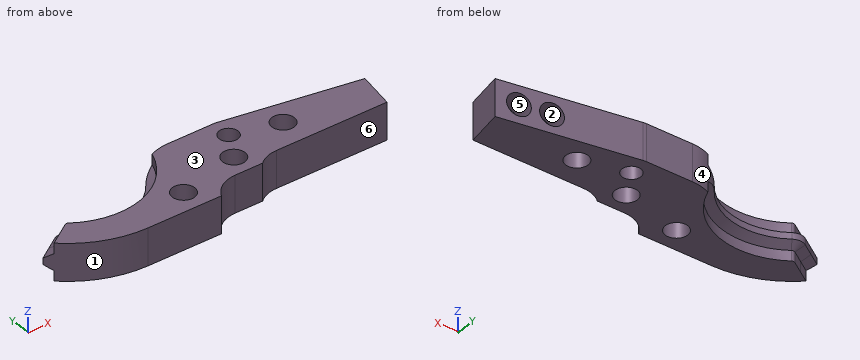
from build123d import *

# Parameters (mm, degrees)
EXTRUDE1_DEPTH                   = 15.621
SKETCH5_W                        = 270.806573858
SKETCH5_H                        = 166.102939791
EXTRUDE2_DEPTH                   = 160.670835286
SKETCH6_R                        = 4
EXTRUDE3_DEPTH                   = 160.670835296
EXTRUDE4_DEPTH                   = 160.670835296
F_3_8_0_375_DIAMETER_HOLE1_D     = 9.525
F_3_8_0_375_DIAMETER_HOLE1_DEPTH = 25.4
F_3_8_0_375_DIAMETER_HOLE1_TIP   = 1.733408241
F_3_8_0_375_DIAMETER_HOLE2_D     = 9.525
F_3_8_0_375_DIAMETER_HOLE2_DEPTH = 9.7639886
F_3_8_0_375_DIAMETER_HOLE2_TIP   = 1.733408241
EXTRUDE7_DEPTH                   = 125.388654342
EXTRUDE7_DEPTH_BACK              = 125.388654342


with BuildPart() as part:
    # Sketch1 → Extrude1 (new body)
    with BuildSketch(Plane.XY):
        with BuildLine():
            Line((-18.523440753, -21.052635779), (-31.956486184, -29.996682998))
            ThreePointArc((-31.956486184, -29.996682998), (-16.785704199, -41.078283404), (1.5875, -45))
            Line((1.5875, -45), (33.100991233, -45))
            ThreePointArc((33.100991233, -45), (37.78291668, -39.890744707), (44.45, -38))
            Line((44.45, -38), (152.4, -38))
            Line((152.4, -38), (152.4, -21.7))
            Line((152.4, -21.7), (139.7, -21.7))
            Line((139.7, -21.7), (139.7, -9))
            Line((139.7, -9), (26.558074677, -9))
            ThreePointArc((26.558074677, -9), (7.242606084, -27.090145582), (-18.523440753, -21.052635779))
        make_face()
    extrude(amount=EXTRUDE1_DEPTH)

    # Cut-Sweep1: sweep along a path in Sketch4
    with BuildLine(Plane.XY.offset(15.621)) as cut_sweep1_path:
        Line((-31.956486184, -29.996682998), (-26.708036397, -26.502137926))
        Line((-26.708036397, -26.502137926), (-21.563139896, -23.076541141))
        ThreePointArc((-21.563139896, -23.076541141), (-18.711510192, -22.22512912), (-15.872310869, -23.117116564))
        ThreePointArc((-15.872310869, -23.117116564), (8.852662428, -26.607549652), (26.558074677, -9))
    # Sketch3 → Cut-Sweep1 (sweep, cut)
    with BuildSketch(Plane(origin=(26.558074677, -9, 15.621), x_dir=(0.9470955536490446, -0.3209517288599796, 0), z_dir=(-0.3209517288599796, -0.9470955536490446, 0))):
        Polygon((-25.4, 0), (3.7084, 0), (3.7084, -4.335954262), (0, -6.477), (0, -9.144), (3.7084, -11.285045738), (3.7084, -15.621), (-25.4, -15.621), (-25.4, -7.8105), align=None)
    sweep(path=cut_sweep1_path.line, mode=Mode.SUBTRACT)

    # Sketch5 → Extrude2 (cut, through all)
    with BuildSketch(Plane.XY.offset(15.621)):
        with Locations((52.123498329, -22.277908904)):
            Rectangle(SKETCH5_W, SKETCH5_H)
        with BuildLine():
            Line((38.333012193, 16.803768596), (31.532220939, 12.275636952))
            ThreePointArc((31.532220939, 12.275636952), (27.554347044, 11.558888171), (24.312391752, 13.972792773))
            ThreePointArc((24.312391752, 13.972792773), (-27.994081927, 1.631780505), (22.524298891, -16.702912621))
            ThreePointArc((22.524298891, -16.702912621), (29.260489218, -11.034352575), (37.826132376, -9))
            Line((37.826132376, -9), (139.7, -9))
            Line((139.7, -9), (139.7, -21.7))
            Line((139.7, -21.7), (152.4, -21.7))
            Line((152.4, -21.7), (152.4, -45))
            Line((152.4, -45), (1.5875, -45))
            ThreePointArc((1.5875, -45), (-37.731008972, 21.887321724), (39.835360247, 23.708673234))
            ThreePointArc((39.835360247, 23.708673234), (40.481466367, 19.95220497), (38.333012193, 16.803768596))
        make_face(mode=Mode.SUBTRACT)
    extrude(amount=-EXTRUDE2_DEPTH, mode=Mode.SUBTRACT)

    # Sketch6 → Extrude3 (cut, through all)
    with BuildSketch(Plane(origin=(0, 0, 0), x_dir=(-1, 0, 0), z_dir=(0, 0, -1))):
        with Locations((-57.5, -17.4625)):
            Circle(SKETCH6_R)
    extrude(amount=-EXTRUDE3_DEPTH, mode=Mode.SUBTRACT)

    # Sketch7 → Extrude4 (cut, through all)
    with BuildSketch(Plane(origin=(0, 0, 0), x_dir=(-1, 0, 0), z_dir=(0, 0, -1))):
        with BuildLine():
            Line((-58.969497704, -9.12856439), (-114.906578075, -18.991780882))
            Line((-114.906578075, -18.991780882), (-110.320627324, -45))
            Line((-110.320627324, -45), (-152.4, -45))
            Line((-152.4, -45), (-152.4, -9))
            Line((-152.4, -9), (-57.5, -9))
            ThreePointArc((-57.5, -9), (-58.237555473, -9.032202367), (-58.969497704, -9.12856439))
        make_face()
    extrude(amount=-EXTRUDE4_DEPTH, mode=Mode.SUBTRACT)

    # 3/8 (0.375) Diameter Hole1
    with Locations(Plane(origin=(0, 0, 0), x_dir=(-1, 0, 0), z_dir=(0, 0, -1))):
        with Locations((-24.181578009, -35.475), (-50.694078075, -29.125), (-76.806578075, -22.775)):
            Hole(F_3_8_0_375_DIAMETER_HOLE1_D / 2, depth=F_3_8_0_375_DIAMETER_HOLE1_DEPTH)
            with Locations((0, 0, -(F_3_8_0_375_DIAMETER_HOLE1_DEPTH + F_3_8_0_375_DIAMETER_HOLE1_TIP / 2))):  # 140° drill point
                Cone(0, F_3_8_0_375_DIAMETER_HOLE1_D / 2, F_3_8_0_375_DIAMETER_HOLE1_TIP, mode=Mode.SUBTRACT)

    # 3/8 (0.375) Diameter Hole2
    with Locations(Plane(origin=(0.217071479, 1.231073535, 0), x_dir=(-0.9848077530122092, 0.17364817766692367, 0), z_dir=(0.17364817766692367, 0.9848077530122092, 0))):
        with Locations((-94.583777101, 7.8105), (-107.283777101, 7.8105)):
            Hole(F_3_8_0_375_DIAMETER_HOLE2_D / 2, depth=F_3_8_0_375_DIAMETER_HOLE2_DEPTH)
            with Locations((0, 0, -(F_3_8_0_375_DIAMETER_HOLE2_DEPTH + F_3_8_0_375_DIAMETER_HOLE2_TIP / 2))):  # 140° drill point
                Cone(0, F_3_8_0_375_DIAMETER_HOLE2_D / 2, F_3_8_0_375_DIAMETER_HOLE2_TIP, mode=Mode.SUBTRACT)

    # Sketch13 → Extrude7 (cut, two sides: drawn at the far end of the back side and taken through both)
    with BuildSketch(Plane.XY.offset(15.621).offset(-EXTRUDE7_DEPTH_BACK)):
        with BuildLine():
            Line((-170.850798283, -238.240416596), (56.200492318, -38))
            ThreePointArc((56.200492318, -38), (60.110624671, -35.645237797), (64.600752731, -34.825))
            Line((64.600752731, -34.825), (112.114754353, -34.825))
            Line((112.114754353, -34.825), (414.849808488, -34.825))
            Line((414.849808488, -34.825), (613.492170854, -606.782396913))
            Line((613.492170854, -606.782396913), (27.791564083, -810.197813509))
            Line((27.791564083, -810.197813509), (-170.850798283, -238.240416596))
        make_face()
    extrude(amount=EXTRUDE7_DEPTH + EXTRUDE7_DEPTH_BACK, mode=Mode.SUBTRACT)


solid = part.part
Build history of the part. All positions in model axes, mm. Face numbers are marked on the shaded views. A direction names the side the tool comes from. Round coordinates to 2 decimals unless told otherwise and drop trailing zeros. Write each loop counter-clockwise with the first axis right and the second up, starting at its lowest first coordinate (ties: lowest second). Pieces come first, ordered by that corner, then holes. Notation, with made-up numbers: M 32.25,-36 L 89.25,-36 A16 cw 89.25,-29 Z; hole C -15.5,-20.75 d8. An arc over 180 degrees is marked long. Answer as a JSON object with one key per item and string values. Group by question number.
(1) Drill centre lines: L1, parallel to X at y = -20.5, z = 9.25; L2, parallel to X at y = -28.5, z = 14; L3, parallel to X at y = -32, z = 14. Where is each one in solid material? Low to high.
(2) Which spindle directions (+Z, -Z, +X, -X, +Y, -Y) get a long thin tool onto all of the face, cutting with end or side? Do the marked faces 5 and 6. Say none if no direction does.
(3) Cut at B-B (x = 31.5). Give the cut face in (y, z).
(4) Cut at A-A (z = 1.75). Give the number of separate pieces and of enclosed holes in the cut face, and give its area (3 significant figures).
(5) Flat gauge pins, fed straight in: pin 1 (3 mm diameter, centred on x = 95.5, z = 8, fed in from -Y) (3 decimals); pin 2 (8 mm diameter, centred on x = 21, y = -17.5, fed in from -Z); pin 3 (8 mm diameter, centred on x = 47.5, z = 14, fed in from -Y). Where does each tip first touch, or does it go through?
(6) Mould opens along Y. For the marked faces 1, 2, 3 and 4 say: pulls with the +Y half, pulls with the -Y half, needs draft (parallel to the pull), parting line crosses it, or undercut.
(7) Cut at C-C (y = -42). Give the cut face in (x, z).
Responses:
{
 "1": {"L1": "x = 19.4 to 54.9, 60.1 to 72.62, 80.99 to 87.82, 97.04 to 100.71, 109.93 to 114.64", "L2": "x = -23.02 to -13.99, 13.99 to 45.97, 55.42 to 113.23", "L3": "x = -28.27 to 20.92, 27.44 to 46.9, 54.49 to 112.61"},
 "2": {"face 5": "none", "face 6": "+Z, -Z, +X, -Y"},
 "3": {"outline": "M -45,0 L -10.08,0 L -10.08,15.62 L -45,15.62 Z"},
 "4": {"separate pieces": "1", "enclosed holes": "4", "area": "2,660 mm2"},
 "5": {"pin 1": "stops at y = -34.825", "pin 2": "stops at z = 4.58", "pin 3": "stops at y = -38.04"},
 "6": {"face 1": "pulls with the -Y half", "face 2": "undercut", "face 3": "needs draft", "face 4": "pulls with the +Y half"},
 "7": {"outline": "M -14.57,0 L 35.2,0 L 35.2,15.62 L -14.57,15.62 Z"}
}
